The model under review builds one solid part; all positions refer to its coordinate system, in mm. A direction names the side the tool comes from. Coordinates: 2 decimals unless noted, no trailing zeros. Write each loop counter-clockwise with the first axis right and the second up, starting at its lowest first coordinate (ties: lowest second). Pieces come first, ordered by that corner, then holes. Notation, with made-up numbers: (-34, 81.25) - (11, 81.25) arc R26 ccw to (11, 112.25) - close; hole circle Ø2 at (12.25, -4.5). An arc over 180 degrees is marked (long way). Return JSON: item names as keys, results as strings. Group by question number.
(1) Tool access review of faces 1 (the face through (-285.75, 0, -49)), 2 (the face through (279.4, 0, 545)): name each direction out of +Z, -Z, +X, -X, +Y, -Y from which nothing blocks a thin tool from reaching the whole face with its end or side.
(2) To check wall thickness, follow L1, parallel to X at y = -6.5, z = -39; L2, parallel to X at y = 8.5, z = 509; L3, parallel to X at y = 4.5, z = 478. State the ranges of each line that lie inside material, in increasing order. Write a range as from..to.
(3) For pin 1 Ø1.5 at (x, y) = (-124, 7) entering from +Z; pin 2 Ø2 at (x, y) = (84.5, 1) entering from +Z (3 decimals); pin 3 Ø9.5 at (x, y) = (-44, -1) entering from +Z, all flat-tipped, find the tip position at first contact; note any pin that passes through.
(4) We need section A-A on z = -116. State the section outline as (x, y) points (3 decimals).
(5) We need section B-B on y = -5.75. Give the number of separate pieces and of enclosed holes in the cut face, then the cut area to 3 significant figures.
```python
from build123d import *

# Parameters (mm, degrees)
F1_DEPTH = 9.525
F2_R     = 25.4
F3_W     = 571.5
F3_H     = 673.1
F4_DEPTH = 19.051
F5_R     = 30.099
F7_DEPTH = 19.051
F8_W     = 571.5
F8_H     = 19.05
F9_DEPTH = 19.05


with BuildPart() as f1:
    # F0 (on Front) → F1 (new body, symmetric)
    with BuildSketch(Plane.XZ):
        Polygon((-304.8, 355.6), (-304.8, -355.6), (304.8, -355.6), (304.8, 355.6), (0, 355.6), align=None)
        Polygon((-304.8, 553.508333), (-304.8, 355.6), (0, 355.6), (-25.4, 373.591667), (-50.8, 373.591667), (-50.8, 391.583333), (-76.2, 391.583333), (-76.2, 409.575), (-101.6, 409.575), (-101.6, 427.566667), (-127, 427.566667), (-127, 445.558333), (-152.4, 445.558333), (-152.4, 463.55), (-177.8, 463.55), (-177.8, 481.541667), (-203.2, 481.541667), (-203.2, 499.533333), (-228.6, 499.533333), (-228.6, 517.525), (-254, 517.525), (-254, 535.516667), (-279.4, 535.516667), (-279.4, 553.508333), align=None)
        Polygon((0, 355.6), (304.8, 355.6), (304.8, 553.508333), (279.4, 553.508333), (279.4, 535.516667), (254, 535.516667), (254, 517.525), (228.6, 517.525), (228.6, 499.533333), (203.2, 499.533333), (203.2, 481.541667), (177.8, 481.541667), (177.8, 463.55), (152.4, 463.55), (152.4, 445.558333), (127, 445.558333), (127, 427.566667), (101.6, 427.566667), (101.6, 409.575), (76.2, 409.575), (76.2, 391.583333), (50.8, 391.583333), (50.8, 373.591667), (25.4, 373.591667), align=None)
    extrude(amount=F1_DEPTH, both=True)

    # F2
    f2_edges = [f1.edges().sort_by_distance(p)[0] for p in [
        (-304.8, 0, -355.6),
        (304.8, 0, -355.6),
    ]]
    fillet(f2_edges, radius=F2_R)

    # F3 (on face) → F4 (cut, through all)
    with BuildSketch(Plane.XZ.offset(9.525)):
        Rectangle(F3_W, F3_H)
    extrude(amount=-F4_DEPTH, mode=Mode.SUBTRACT)

    # F5
    f5_edges = [f1.edges().sort_by_distance(p)[0] for p in [
        (285.75, 0, -336.55),
        (-285.75, 0, -336.55),
    ]]
    fillet(f5_edges, radius=F5_R)

    # F6 (on face) → F7 (cut, through all)
    with BuildSketch(Plane.XZ.offset(9.525)):
        Polygon((-285.75, 355.6), (-105.537, 355.6), (-285.75, 517.525), align=None)
        Polygon((105.526209, 355.6), (285.75, 355.6), (285.75, 517.525), align=None)
    extrude(amount=-F7_DEPTH, mode=Mode.SUBTRACT)

    # F8 (on face) → F9 (join)
    with BuildSketch(Plane.XZ.offset(9.525)):
        with Locations((0, 164.465)):
            Rectangle(F8_W, F8_H)
        with Locations((0, 249.555)):
            Rectangle(F8_W, F8_H)
        with Locations((0, 79.375)):
            Rectangle(F8_W, F8_H)
        with Locations((0, -5.715)):
            Rectangle(F8_W, F8_H)
        with Locations((0, -90.805)):
            Rectangle(F8_W, F8_H)
        with Locations((0, -175.895)):
            Rectangle(F8_W, F8_H)
        with Locations((0, -260.985)):
            Rectangle(F8_W, F8_H)
    extrude(amount=-F9_DEPTH)


solid = f1.part
```
Ans:
{
 "1": {"face 1": "+Y, -Y", "face 2": "+Z, +Y, -Y"},
 "2": {"L1": "-304.8..-285.75, 285.75..304.8", "L2": "-304.8..-285.75, -276.26..-228.6, 228.6..276.26, 285.75..304.8", "L3": "-304.8..-285.75, -241.76..-177.8, 177.8..241.76, 285.75..304.8"},
 "3": {"pin 1": "z = 427.57", "pin 2": "z = 409.575", "pin 3": "z = 373.59"},
 "4": {"outline": "(-304.8, -9.525) - (-285.75, -9.525) - (-285.75, 9.525) - (-304.8, 9.525) - close; (285.75, -9.525) - (304.8, -9.525) - (304.8, 9.525) - (285.75, 9.525) - close"},
 "5": {"separate pieces": "1", "enclosed holes": "10", "area": "157,000 mm²"}
}
